Check sheet for the modelled part. Datum: model origin and axes. Units: mm. Face numbers are marked on the shaded views. A direction names the side the tool comes from. Give positions to 0.01 mm unless a question says otherwise; leave off trailing zeros. Order: outer loops, then holes, each group sorted by start corner. A loop starts at its lowest first (then second) coordinate and runs counter-clockwise, first axis right, second up. Notation, with made-up numbers: M 32,-31.5 L 86,-31.5 A26 cw 86,-7.5 Z; hole C 64,30 d2. An arc over 180 degrees is marked long. Answer in a Markdown table with one row per item. Add a question column.
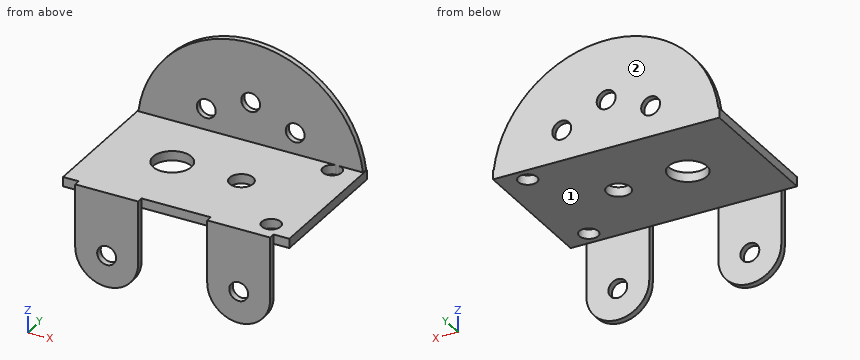
from build123d import *

# Parameters (mm, degrees)
CROQUIS1_W              = 36
CROQUIS1_H              = 22.25
CROQUIS1_R              = 1.5
CROQUIS1_R_2            = 3.05
CROQUIS1_R_3            = 1.875
SALIENTE_EXTRUIR1_DEPTH = 1.5
CROQUIS2_R              = 1.5
CROQUIS2_W              = 10
CROQUIS2_H              = 1.5
SALIENTE_EXTRUIR2_DEPTH = 1
CROQUIS3_R              = 1.500000001
CROQUIS3_R_2            = 1.5
SALIENTE_EXTRUIR6_DEPTH = 0.9


with BuildPart() as part:
    # Croquis1 → Saliente-Extruir1 (new body)
    with BuildSketch(Plane.XY):
        Rectangle(CROQUIS1_W, CROQUIS1_H)
        with Locations((13.8, 8.745)):
            Circle(CROQUIS1_R, mode=Mode.SUBTRACT)
        with Locations((-6.8, 0)):
            Circle(CROQUIS1_R_2, mode=Mode.SUBTRACT)
        with Locations(Location((13.8, -8.745, 0), (0, 0, 180))):
            Circle(CROQUIS1_R, mode=Mode.SUBTRACT)
        with Locations((4.2, 0)):
            Circle(CROQUIS1_R_3, mode=Mode.SUBTRACT)
    extrude(amount=SALIENTE_EXTRUIR1_DEPTH)

    # Croquis2 → Saliente-Extruir2 (add)
    # profile 1 of 4: a face of its own
    with BuildSketch(Plane.XZ.offset(11.125)):
        with BuildLine():
            Line((-5.5, -8.5), (-5.5, 0))
            Line((-5.5, 0), (-15.5, 0))
            Line((-15.5, 0), (-15.5, -8.5))
            ThreePointArc((-15.5, -8.5), (-10.5, -13.5), (-5.5, -8.5))
        make_face()
        with Locations((-10.5, -8.5)):
            Circle(CROQUIS2_R, mode=Mode.SUBTRACT)
    # profile 2 of 4: a face of its own
    with BuildSketch(Plane.XZ.offset(11.125)):
        with Locations((-10.5, 0.75)):
            Rectangle(CROQUIS2_W, CROQUIS2_H)
    # profile 3 of 4: a face of its own
    with BuildSketch(Plane.XZ.offset(11.125)):
        with BuildLine():
            Line((15.5, 0), (5.5, 0))
            Line((5.5, 0), (5.5, -8.5))
            ThreePointArc((5.5, -8.5), (10.5, -13.5), (15.5, -8.5))
            Line((15.5, -8.5), (15.5, 0))
        make_face()
        with Locations((10.5, -8.5)):
            Circle(CROQUIS2_R, mode=Mode.SUBTRACT)
    # profile 4 of 4: a face of its own
    with BuildSketch(Plane.XZ.offset(11.125)):
        with Locations((10.5, 0.75)):
            Rectangle(CROQUIS2_W, CROQUIS2_H)
    extrude(amount=SALIENTE_EXTRUIR2_DEPTH)

    # Croquis3 → Saliente-Extruir6 (add)
    # profile 1 of 2: a face of its own
    with BuildSketch(Plane(origin=(0, 11.125, 0), x_dir=(1, 0, 0), z_dir=(0, 1, 0))):
        with BuildLine():
            ThreePointArc((-17.865049678, -1.5), (0, -17.3), (17.865049678, -1.5))
            Line((17.865049678, -1.5), (-17.865049678, -1.5))
        make_face()
        with Locations(Location((-7.071067812, -4.871067812, 0), (0, 0, 180))):
            Circle(CROQUIS3_R, mode=Mode.SUBTRACT)
        with Locations(Location((0, -7.8, 0), (0, 0, 180))):
            Circle(CROQUIS3_R_2, mode=Mode.SUBTRACT)
        with Locations(Location((7.071067812, -4.871067812, 0), (0, 0, 180))):
            Circle(CROQUIS3_R_2, mode=Mode.SUBTRACT)
    # profile 2 of 2: a face of its own
    with BuildSketch(Plane(origin=(0, 11.125, 0), x_dir=(1, 0, 0), z_dir=(0, 1, 0))):
        with BuildLine():
            ThreePointArc((17.865049678, -1.5), (17.941399597, -0.751268579), (17.986383739, 0))
            Line((17.986383739, 0), (-17.986383739, 0))
            ThreePointArc((-17.986383739, 0), (-17.941399597, -0.751268579), (-17.865049678, -1.5))
            Line((-17.865049678, -1.5), (17.865049678, -1.5))
        make_face()
    extrude(amount=-SALIENTE_EXTRUIR6_DEPTH)


solid = part.part
Q1. Cross-section at D-D (z = 1). Record the boundary of the cut face in (x, y) (3 decimals).
Q2. Thickness scan on probe 1 along Y at (x, z) = (13.8, 0.75) (3 decimals); probe 2 along Z at (x, y) = (10.5, -11.65); probe 3 along Z at (x, y) = (0, 10.7). Record the ranges inside material, lowest first.
Q3. Cross-section at A-A (y = 0). Record the boundary of the cut face in (x, z) (3 decimals).
Q4. Go/stop test with flat-tipped pins: pin 1 (4 mm diameter, centred on x = 13.8, y = -8.745, fed in from +Z); pin 2 (5 mm diameter, centred on x = 7.07, z = 4.87, fed in from -Y) (3 decimals); pin 3 (8 mm diameter, centred on x = -8.5, z = -9.5, fed in from +Y) (3 decimals). Record where each tip stops, or that it passes through.
Q5. Cross-section at B-B (x = 0). Record the boundary of the cut face in (y, z) (3 decimals).
Q6. Cross-section at C-C (y = 2.5). Record the boundary of the cut face in (x, z).
Q7. Tool access check on the marked faces 1 and 2. Record the directions out of +Z, -Z, +X, -X, +Y, -Y that give a thin tool (end or side, any length) a straight path to the whole face; none if there is none.
Values follow:
| question | item | result |
|---|---|---|
| 1 | outline | M -18,-11.125 L -15.5,-11.125 L -15.5,-12.125 L -5.5,-12.125 L -5.5,-11.125 L 5.5,-11.125 L 5.5,-12.125 L 15.5,-12.125 L 15.5,-11.125 L 18,-11.125 L 18,11.125 L -18,11.125 Z; hole C -6.8,0 d6.1; hole C 4.2,0 d3.75; hole C 13.8,-8.745 d3; hole M 13.556,10.225 A1.5 ccw long 14.044,10.225 Z |
| 2 | probe 1 | -12.125 to -10.245, -7.245 to 7.245, 10.225 to 11.125 |
| 2 | probe 2 | -13.5 to -10, -7 to 1.5 |
| 2 | probe 3 | 0 to 6.3, 9.3 to 17.3 |
| 3 | outline | M -18,0 L -9.85,0 L -9.85,1.5 L -18,1.5 Z; M -3.75,0 L 2.325,0 L 2.325,1.5 L -3.75,1.5 Z; M 6.075,0 L 18,0 L 18,1.5 L 6.075,1.5 Z |
| 4 | pin 1 | z = 1.5 |
| 4 | pin 2 | y = 10.225 |
| 4 | pin 3 | y = -11.125 |
| 5 | outline | M -11.125,0 L 11.125,0 L 11.125,6.3 L 10.225,6.3 L 10.225,1.5 L -11.125,1.5 Z; M 10.225,9.3 L 11.125,9.3 L 11.125,17.3 L 10.225,17.3 Z |
| 6 | outline | M -18,0 L -8.55,0 L -8.55,1.5 L -18,1.5 Z; M -5.05,0 L 18,0 L 18,1.5 L -5.05,1.5 Z |
| 7 | face 1 | -Z, +X, -X, +Y |
| 7 | face 2 | +Z, -Z, +X, -X, +Y |
